```python
from build123d import *

# Parameters (mm, degrees)
SKETCH_1_R = 1
PCB_DEPTH  = 1.6
XT60_DEPTH = 16
XT30_DEPTH = 10.7
FILLET_2_R = 1


with BuildPart() as part:
    # 草图1 → PCB (new body)
    with BuildSketch(Plane(origin=(0, 0, 0), x_dir=(1, 0, 0), z_dir=(0, 1, 0))):
        Polygon((-26.5, 17.5), (-21.5, 23.5), (-11.5, 23.5), (-6.5, 17.5), (6.5, 17.5), (11.5, 23.5), (21.5, 23.5), (26.5, 17.5), (41.5, 17.5), (41.5, 7.5), (46.5, 7.5), (46.5, -7.5), (41.5, -7.5), (41.5, -17.5), (26.5, -17.5), (21.5, -23.5), (11.5, -23.5), (6.5, -17.5), (-6.5, -17.5), (-11.5, -23.5), (-21.5, -23.5), (-26.5, -17.5), (-41.5, -17.5), (-41.5, -7.5), (-46.5, -7.5), (-46.5, 7.5), (-41.5, 7.5), (-41.5, 17.5), align=None)
        with Locations((-39.5, 15.5)):
            Circle(SKETCH_1_R, mode=Mode.SUBTRACT)
        with Locations((-39.5, -15.5)):
            Circle(SKETCH_1_R, mode=Mode.SUBTRACT)
        with Locations((39.5, -15.5)):
            Circle(SKETCH_1_R, mode=Mode.SUBTRACT)
        with Locations((39.5, 15.5)):
            Circle(SKETCH_1_R, mode=Mode.SUBTRACT)
    extrude(amount=PCB_DEPTH)

    # 草图3 → XT60 (add)
    with BuildSketch(Plane(origin=(0, 1.6, 0), x_dir=(1, 0, 0), z_dir=(0, 1, 0))):
        Polygon((28.95, 5.45), (31.5, 8), (34.5, 8), (37.05, 5.45), (37.05, -8), (28.95, -8), align=None)
    extrude(amount=XT60_DEPTH)

    # 草图4 → XT30 (add)
    with BuildSketch(Plane(origin=(0, 1.6, 0), x_dir=(1, 0, 0), z_dir=(0, 1, 0))):
        Polygon((-34.4, 5.1), (-35.8, 3.7), (-35.8, -5.1), (-30.2, -5.1), (-30.2, 3.7), (-31.6, 5.1), align=None)
    extrude(amount=XT30_DEPTH)

    # 圆角2
    fillet_2_edges = [part.edges().sort_by_distance(p)[0] for p in [
        (46.5, 0.8, -7.5),
        (46.5, 0.8, 7.5),
        (41.5, 0.8, 17.5),
        (21.5, 0.8, 23.5),
        (11.5, 0.8, 23.5),
        (-11.5, 0.8, 23.5),
        (-21.5, 0.8, 23.5),
        (-41.5, 0.8, 17.5),
        (-46.5, 0.8, 7.5),
        (-46.5, 0.8, -7.5),
        (-41.5, 0.8, -17.5),
        (-21.5, 0.8, -23.5),
        (-11.5, 0.8, -23.5),
        (11.5, 0.8, -23.5),
        (21.5, 0.8, -23.5),
        (41.5, 0.8, -17.5),
    ]]
    fillet(fillet_2_edges, radius=FILLET_2_R)


solid = part.part
```
Could you check a few things on this model? Use its own coordinates, in mm. A direction names the side the tool comes from. Round coordinates to 2 decimals unless told otherwise and drop trailing zeros. Loops run counter-clockwise (first coordinate to the right, second up) from the corner with the lowest first, then second, coordinate; pieces in that order, holes last. Notation, with made-up numbers: (-21.5, -25.5) - (27.5, -25.5) arc R20 ccw to (27.5, 8.5) - close; hole circle Ø5 at (48, -2.75). An arc over 180 degrees is marked (long way). Answer in a Markdown table with one row per item. Add a question column.
(1) For faces 5 (the face through (30.2, 9.5, -6.7)), 6 (the face through (44, 1, 7.5)), 7 (the face through (28.95, 9, 1)), 8 (the face through (33, 9, 8)), 9 (the face through (35.8, 9.5, -6.7)), which set-ups out of +Z, -Z, +X, -X, +Y, -Y let a thin tool reach every point of the face, with its end or its side?
(2) If we section it at C-C (z = -15.5): Please give me the cut outline in (x, y).
(3) I need wall thicknesses on line 1 along Z through (x, y) = (39.5, 1.1); line 2 along X through (y, z) = (0.9, 15.5); line 3 along X through (y, z) = (10.5, 1). Which ranges of each line are inside material? Lowest first, please.
(4) If we section it at B-B (y = 6.75): Please give me the cut outline in (x, z).
(5) I'm going to push flat-ended pins straight in: pin 1 (5 mm diameter, centred on x = -12.5, z = -6.5, fed in from +Y); pin 2 (0.8 mm diameter, centred on y = 1, z = 10.5, fed in from +X); pin 3 (4.5 mm diameter, centred on x = -33, y = 5.5, fed in from +Z); pin 4 (8 mm diameter, centred on y = 7, z = -17.5, fed in from -X). Where does each tip first touch, or does it pass through?
(6) If we section it at A-A (x = -39.5): Please give me the cut outline in (y, z).
(7) If we mould it in two halves opening along X, with no side actions, what happens to faces 1 (the face through (-39.04, 0.79, 16.39)), 2 (the face through (41.5, 1, -12)), 3 (the face through (-34, 1, -17.5)), 4 (the face through (-8.883, 0.789, -20.36))? For each: pulls with the +X half, pulls with the -X half, needs draft (parallel to the pull), parting line crosses it, or undercut.
(8) If we section it at D-D (y = 16): Please give me the cut outline in (x, z), plus the area to 3 significant figures.
Model answer:
| question | item | result |
|---|---|---|
| 1 | face 5 | -Z, -X, +Y |
| 1 | face 6 | +Z, +X, +Y, -Y |
| 1 | face 7 | +Z, -Z, +Y |
| 1 | face 8 | +Z, +X, -X, +Y |
| 1 | face 9 | -Z, +X, +Y |
| 2 | outline | (-41.5, 0) - (-40.5, 0) - (-40.5, 1.6) - (-41.5, 1.6) - close; (-38.5, 0) - (38.5, 0) - (38.5, 1.6) - (-38.5, 1.6) - close; (40.5, 0) - (41.5, 0) - (41.5, 1.6) - (40.5, 1.6) - close |
| 3 | line 1 | z = -17.5 to -16.5, -14.5 to 14.5, 16.5 to 17.5 |
| 3 | line 2 | x = -41.5 to -40.5, -38.5 to 38.5, 40.5 to 41.5 |
| 3 | line 3 | x = -35.8 to -30.2, 28.95 to 37.05 |
| 4 | outline | (-35.8, -3.7) - (-34.4, -5.1) - (-31.6, -5.1) - (-30.2, -3.7) - (-30.2, 5.1) - (-35.8, 5.1) - close; (28.95, -5.45) - (31.5, -8) - (34.5, -8) - (37.05, -5.45) - (37.05, 8) - (28.95, 8) - close |
| 5 | pin 1 | stops at y = 1.6 |
| 5 | pin 2 | stops at x = 41.5 |
| 5 | pin 3 | stops at z = 5.1 |
| 5 | pin 4 | passes through |
| 6 | outline | (0, -17.5) - (1.6, -17.5) - (1.6, -16.5) - (0, -16.5) - close; (0, -14.5) - (1.6, -14.5) - (1.6, 14.5) - (0, 14.5) - close; (0, 16.5) - (1.6, 16.5) - (1.6, 17.5) - (0, 17.5) - close |
| 7 | face 1 | undercut |
| 7 | face 2 | pulls with the +X half |
| 7 | face 3 | needs draft |
| 7 | face 4 | undercut |
| 8 | outline | (28.95, -5.45) - (31.5, -8) - (34.5, -8) - (37.05, -5.45) - (37.05, 8) - (28.95, 8) - close |
| 8 | area | 123 mm² |
